Verification items for the finished model (mm, model axes). Face numbers are marked on the shaded views. A direction names the side the tool comes from. Give positions to 0.01 mm unless a question says otherwise; leave off trailing zeros. Loops run counter-clockwise (first coordinate to the right, second up) from the corner with the lowest first, then second, coordinate; pieces in that order, holes last. Notation, with made-up numbers: (-2, 80) - (18, 80) arc R12 ccw to (18, 85) - close; hole circle Ø8 at (49.5, -30). An arc over 180 degrees is marked (long way). Answer in a Markdown table with one row per item.
Autodesk Inventor part; units mm, degrees
ref_plane "Work Plane1" through (-5, 0, 0) normal (1, 0, 0) x (0, 1, 0)
ref_plane "Work Plane2" through (-7, 0, 0) normal (1, 0, 0) x (0, 1, 0)
ref_plane "XZ Plane" through (0, 0, 0) normal (0, 1, 0) x (-1, 0, 0)
sketch "Sketch1" plane through (0, 0, 0) normal (0, 1, 0) x (-1, 0, 0)
  circle A0 centre (0, 0) radius 2.35
  circle A1 centre (0, 0) radius 5
  circle A2 centre (-10, 0) radius 1.5
  line L0 (-0.75, 4.9434) -> (-10.525, 3.4604)
  arc A3 (-10.525, 3.4604) -> (-10.525, -3.4604) centre (-10, 0) ccw
  line L1 (-10.525, -3.4604) -> (-0.75, -4.9434)
  dimension "d0" = 4.7
  dimension "d1" = 10
  dimension "d2" = 3
  dimension "d3" = 10
  dimension "d4" = 2
extrude "Extrusion1" add sketch "Sketch1" against normal blind 2 and the other way blind 2 contours A0 | A1 | A1 L1 A3 L0
extrude "Extrusion2" add sketch "Sketch1" along normal blind 30 contours A1
extrude "Extrusion3" add sketch "Sketch1" along normal blind 32 contours A0
ref_plane "Work Plane1" through (-5, 0, 0) normal (1, 0, 0) x (0, 1, 0)
ref_plane "Work Plane2" through (-7, 0, 0) normal (1, 0, 0) x (0, 1, 0)
sketch "Sketch2" plane through (-7, 0, 0) normal (1, 0, 0) x (0, 1, 0)
  line L0 (30, -15) -> (-2, -15)
  line L1 (-2, 15) -> (30, 15)
  line L2 (30, 15) -> (30, -15)
  line L3 (30, -5) -> (30, 5)
  line L4 (-2, -4.9434) -> (2, -4.9434)
  line L5 (-2, 4.9434) -> (-2, -4.9434)
  line L6 (2, 4.9434) -> (-2, 4.9434)
  line L7 (2, -4.9434) -> (2, 4.9434)
  line L8 (-2, -15) -> (-2, 15)
  point P0 (0, 0)
  dimension "d11" = 30
  dimension "d12" = 15
sketch "Sketch3" plane through (-7, 0, 0) normal (-1, 0, 0) x (0, 0, 1)
  line L0 (-10, 22.6542) -> (10, 22.6542) construction
  line L1 (10, 22.6542) -> (10, 2.6542) construction
  line L2 (10, 2.6542) -> (-10, 2.6542) construction
  line L3 (-10, 2.6542) -> (-10, 22.6542) construction
  line L4 (15, -2) -> (15, 30) construction
  line L5 (15, 30) -> (-15, 30) construction
  line L6 (0, 0) -> (15, 0) construction
  point P0 (0, 0)
  point P1 (10, 12.6542)
  point P2 (15, 14)
  point P3 (0, 22.6542)
  point P4 (0, 30)
  dimension "d24" = 20
  dimension "d25" = 20
properties part number "Pok Mk3 Yaw Motor Support Min" material "ABS Plastic"
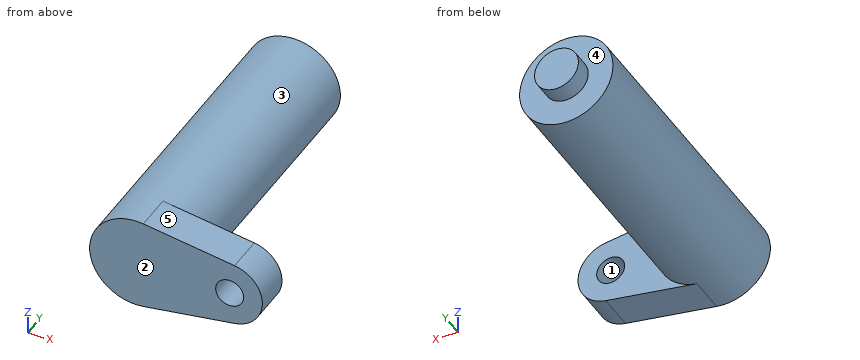
Q1. Sectioned sample at A-A (y = 1.5). Record the cut outline in (x, z) (3 decimals), and give its area (3 significant figures).
Completed:
| item | result |
|---|---|
| outline | (0.75, -4.943) - (10.525, -3.46) arc R3.5 ccw to (10.525, 3.46) - (0.75, 4.943) arc R5 ccw (long way) to start; hole circle Ø3 at (10, 0) |
| area | 137 mm^2 |
Q2. Sectioned sample at B-B (x = 10). Record the cut outline in (y, z), and give its area (3 significant figures).
Completed:
| item | result |
|---|---|
| outline | (-2, -3.54) - (2, -3.54) - (2, -1.5) - (-2, -1.5) - close; (-2, 1.5) - (2, 1.5) - (2, 3.54) - (-2, 3.54) - close |
| area | 16.3 mm^2 |
Q3. Go/stop test with flat-tipped pins: P1, Ø5, axis at x = 9, z = 2.5, coming from the +Y side; P2, Ø1.5, axis at y = 17.5, z = 0.5, coming from the +X side; P3, Ø3, axis at y = 22, z = 3.5, coming from the -X side. Record where each tip stops, or that it passes through.
Completed:
| item | result |
|---|---|
| P1 | y = 2 |
| P2 | x = 5 |
| P3 | x = -4.58 |
Q4. Draft check along X on the marked faces 1, 2 and 3. Enter one of: +X half, -X half, draft (parallel to the pull), parting line (faces both ways), or undercut.
Completed:
| item | result |
|---|---|
| face 1 | undercut |
| face 2 | draft |
| face 3 | parting line |
Q5. Tool access check on the marked faces 4 and 5. Record the directions out of +Z, -Z, +X, -X, +Y, -Y that give a thin tool (end or side, any length) a straight path to the whole face; none if there is none.
Completed:
| item | result |
|---|---|
| face 4 | +Y |
| face 5 | +Z, +X, +Y, -Y |
Q6. Sectioned sample at D-D (y = 28.5). Record the cut outline in (x, z).
Completed:
| item | result |
|---|---|
| outline | circle Ø10 at (0, 0) |
Q7. Sectioned sample at C-C (z = -2). Record the cut outline in (x, y).
Completed:
| item | result |
|---|---|
| outline | (-4.58, -2) - (12.87, -2) - (12.87, 2) - (4.58, 2) - (4.58, 30) - (1.23, 30) - (1.23, 32) - (-1.23, 32) - (-1.23, 30) - (-4.58, 30) - close |
Q8. Thickness scan on line 1 (Y direction, x = 0, z = 2.75); line 2 (Z direction, x = 10, y = 0.65); line 3 (Y direction, x = 11.25, z = -2.5). Record the ranges inside material, lowest first.
Completed:
| item | result |
|---|---|
| line 1 | -2 to 30 |
| line 2 | -3.54 to -1.5, 1.5 to 3.54 |
| line 3 | -2 to 2 |
